The figure shows three views and two pictorial views of one solid part (mm, origin at its lowest corner). Answer the questions. A direction names the side the tool comes from. Round coordinates to 2 decimals unless told otherwise and drop trailing zeros. Order: outer loops, then holes, each group sorted by start corner. A loop starts at its lowest first (then second) coordinate and runs counter-clockwise, first axis right, second up. Notation, with made-up numbers: M 50.25,-36.75 L 75.25,-36.75 A30 cw 75.25,-3.75 Z; hole C 83,60 d9. An arc over 180 degrees is marked long. Answer as CSV lines item,"result".
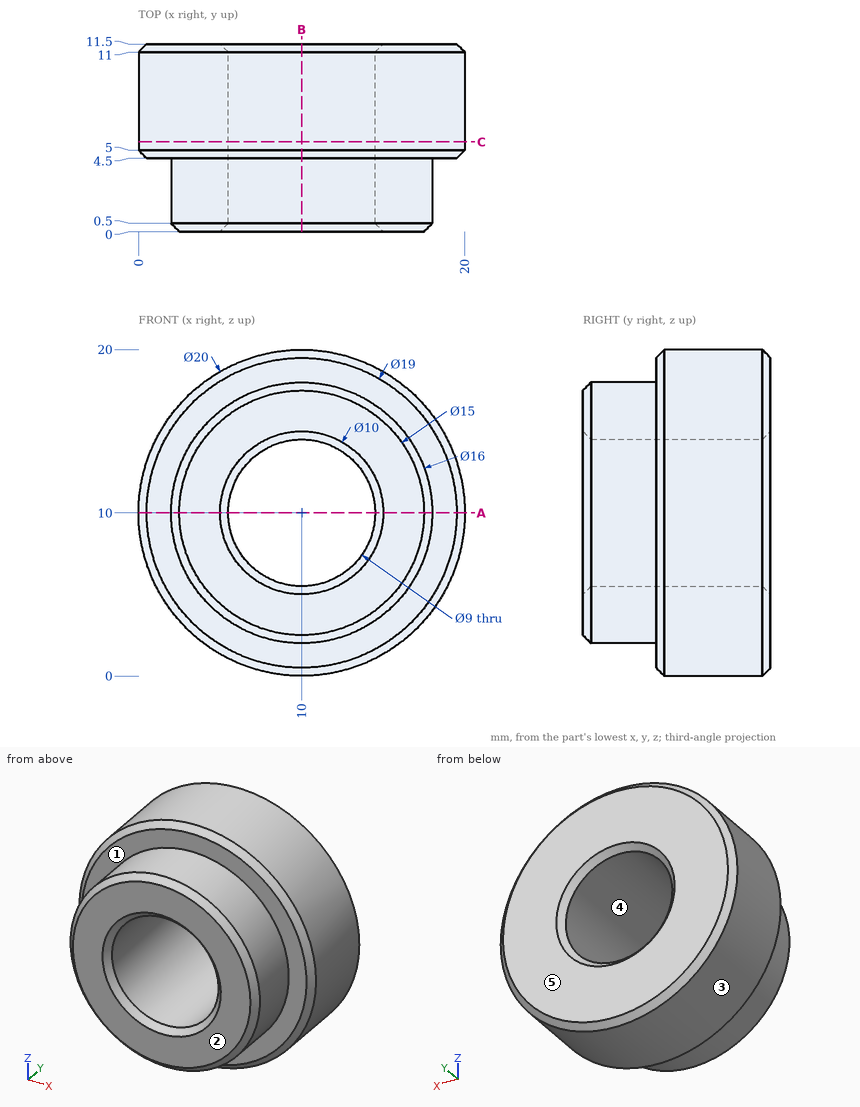
Item 1: Find the intervals of material crossed by probe 1 along X at (y, z) = (3.25, 10); probe 2 along Y at (x, z) = (1.75, 8); probe 3 along Z at (x, y) = (4, 10.5), in increasing order. Write a range as [from, to].
Ans:
probe 1,"[2, 5.5], [14.5, 18]"
probe 2,"[4.5, 11.5]"
probe 3,"[2, 18]"
Item 2: A tool of negligible diameter and unlimited length cuts with its end or side. For the marked faces 1 and 2, from which of +Z, -Z, +X, -X, +Y, -Y can it reach the whole face along a straight path? Write none if from no direction.
Ans:
face 1,"-Y"
face 2,"+Z, -Z, +X, -X, -Y"
Item 3: A cutting plane is placed at C-C, the plane y = 5.5. Determine the outline of the cut face in (x, z), and give its area (3 significant figures).
Ans:
outline,"C 10,10 d20; hole C 10,10 d9"
area,"251 mm2"
Item 4: Determine the mould class of the marked faces 3, 4 and 5 for opening direction X: +X half, -X half, draft (parallel to the pull), parting line (faces both ways), or undercut.
Ans:
face 3,"parting line"
face 4,"undercut"
face 5,"draft"
Item 5: A cutting plane is placed at A-A, the plane z = 10. Determine the outline of the cut face in (x, y), and give its area (3 significant figures).
Ans:
outline,"M 0,5 L 0.5,4.5 L 2,4.5 L 2,0.5 L 2.5,0 L 5,0 L 5.5,0.5 L 5.5,11 L 5,11.5 L 0.5,11.5 L 0,11 Z; M 14.5,0.5 L 15,0 L 17.5,0 L 18,0.5 L 18,4.5 L 19.5,4.5 L 20,5 L 20,11 L 19.5,11.5 L 15,11.5 L 14.5,11 Z"
area,"107 mm2"
Item 6: Flat-ended cylindrical pins translate along their axes: pin 1 (5 mm diameter, centred on x = 17, y = 6, fed in from -Z); pin 2 (1 mm diameter, centred on y = 6.5, z = 4.5, fed in from -X); pin 3 (9.5 mm diameter, centred on x = 5.5, z = 7.5, fed in from -Y); pin 4 (2 mm diameter, centred on y = 2.5, z = 9, fed in from -X). Find the tip coordinate at first contact, or state that the pin passes through.
Ans:
pin 1,"z = 1.07"
pin 2,"x = 1.34"
pin 3,"y = 0"
pin 4,"x = 2"
Item 7: A cutting plane is placed at B-B, the plane x = 10. Determine the outline of the cut face in (y, z), and give its area (3 significant figures).
Ans:
outline,"M 0,2.5 L 0.5,2 L 4.5,2 L 4.5,0.5 L 5,0 L 11,0 L 11.5,0.5 L 11.5,5 L 11,5.5 L 0.5,5.5 L 0,5 Z; M 0,15 L 0.5,14.5 L 11,14.5 L 11.5,15 L 11.5,19.5 L 11,20 L 5,20 L 4.5,19.5 L 4.5,18 L 0.5,18 L 0,17.5 Z"
area,"107 mm2"
